Autodesk Inventor part; units mm, degrees
ref_plane "YZ Plane" through (0, 0, 0) normal (1, 0, 0) x (0, 1, 0)
ref_plane "XZ Plane" through (0, 0, 0) normal (0, 1, 0) x (-1, 0, 0)
ref_plane "XY Plane" through (0, 0, 0) normal (0, 0, 1) x (1, 0, 0)
sketch "Sketch1" plane through (0, 0, 0) normal (0, 1, 0) x (-1, 0, 0)
  line L0 (0, 0) -> (33, 0)
  line L1 (33, 0) -> (33, -28)
  line L2 (33, -28) -> (0, -28)
  line L3 (0, -28) -> (0, 0)
  line L4 (0, -17.5) -> (-20, -17.5)
  line L5 (-20, -17.5) -> (-20, -10.5)
  line L6 (-20, -10.5) -> (0, -10.5)
  line L7 (0, -10.5) -> (0, -17.5)
  line L8 (33, -17.5) -> (53, -17.5)
  line L9 (53, -17.5) -> (53, -10.5)
  line L10 (53, -10.5) -> (33, -10.5)
  line L11 (33, -10.5) -> (33, -17.5)
  line L12 (20, -28) -> (13, -28)
  line L13 (13, -28) -> (13, -48)
  line L14 (13, -48) -> (20, -48)
  line L15 (20, -48) -> (20, -28)
  line L16 (20, 0) -> (13, 0)
  line L17 (13, 0) -> (13, 20)
  line L18 (13, 20) -> (20, 20)
  line L19 (20, 20) -> (20, 0)
  circle A0 centre (16.5, -44) radius 1.75
  circle A1 centre (-16, -14) radius 1.75
  circle A2 centre (16.5, 16) radius 1.75
  circle A3 centre (49, -14) radius 1.75
  line L20 (16.5, -44) -> (16.5, -48) construction
  line L21 (-16, -14) -> (-20, -14) construction
  line L22 (16.5, 16) -> (16.5, 20) construction
  line L23 (49, -14) -> (53, -14) construction
  circle A4 centre (43, -14) radius 1.75
  circle A5 centre (37, -14) radius 1.75
  circle A6 centre (16.5, -38) radius 1.75
  circle A7 centre (16.5, -32) radius 1.75
  circle A8 centre (-10, -14) radius 1.75
  circle A9 centre (-4, -14) radius 1.75
  circle A10 centre (16.5, 10) radius 1.75
  circle A11 centre (16.5, 4) radius 1.75
  point P0 (16.5, -28)
  point P1 (16.5, 0)
  point P2 (0, -14)
  point P3 (33, -14)
  dimension "d0" = 33
  dimension "d1" = 28
  dimension "d29" = 7
  dimension "d34" = 20
  dimension "d35" = 4
  dimension "d36" = 3.5
  dimension "d44" = 6
  dimension "d51" = 6
  dimension "d58" = 6
  dimension "d65" = 6
extrude "Extrusion1" add sketch "Sketch1" along normal blind 2
sketch "Sketch2" plane through (0, 2, 0) normal (0, 1, 0) x (1, 0, 0)
  line L0 (0, 28) -> (-13, 28)
  line L1 (-33, 28) -> (-33, 17.5)
  line L2 (-33, 0) -> (-20, 0)
  line L3 (0, 0) -> (0, 10.5)
  line L4 (-26.6, 1.85) -> (-6.4, 1.85)
  line L5 (-6.4, 1.85) -> (-6.4, 4.05)
  line L6 (-6.4, 4.05) -> (-26.6, 4.05)
  line L7 (-26.6, 4.05) -> (-26.6, 1.85)
  line L8 (-26.6, 23.95) -> (-6.4, 23.95)
  line L9 (-6.4, 23.95) -> (-6.4, 26.15)
  line L10 (-6.4, 26.15) -> (-26.6, 26.15)
  line L11 (-26.6, 26.15) -> (-26.6, 23.95)
  line L12 (-26.6, 1.85) -> (-33, 1.85)
  line L13 (-26.6, 1.85) -> (-26.6, 0)
  line L14 (-26.6, 26.15) -> (-26.6, 28)
  line L15 (-6.4, 4.05) -> (0, 4.05)
  line L16 (-13, 28) -> (-13, 48)
  line L17 (-13, 48) -> (-20, 48)
  line L18 (-20, 48) -> (-20, 28)
  line L19 (-20, 28) -> (-33, 28)
  line L20 (-33, 17.5) -> (-53, 17.5)
  line L21 (-53, 17.5) -> (-53, 10.5)
  line L22 (-53, 10.5) -> (-33, 10.5)
  line L23 (-33, 10.5) -> (-33, 0)
  line L24 (-20, 0) -> (-20, -20)
  line L25 (-20, -20) -> (-13, -20)
  line L26 (-13, -20) -> (-13, 0)
  line L27 (-13, 0) -> (0, 0)
  line L28 (0, 10.5) -> (20, 10.5)
  line L29 (20, 10.5) -> (20, 17.5)
  line L30 (20, 17.5) -> (0, 17.5)
  line L31 (0, 17.5) -> (0, 28)
  line L32 (-28.5, 21.5) -> (-4.5, 21.5)
  line L33 (-4.5, 21.5) -> (-4.5, 6.5)
  line L34 (-4.5, 6.5) -> (-28.5, 6.5)
  line L35 (-28.5, 6.5) -> (-28.5, 21.5)
  line L36 (-28.5, 21.5) -> (-4.5, 6.5) construction
  line L37 (-4.5, 21.5) -> (-28.5, 6.5) construction
  point P0 (-16.5, 14)
  point P1 (-16.5, 23.95)
  point P2 (20, 14)
  dimension "d4" = 2.2
  dimension "d5" = 20.2
  dimension "d6" = 19.9
  dimension "d37" = 24
  dimension "d38" = 15
extrude "Extrusion2" cut sketch "Sketch2" against normal through all contours L10 L9 L8 L11 | L5 L4 L7 L6 | L32 L33 L34 L35
fillet "Fillet1" radius 3.5 8 edges at (-20, 1, 20) (-13, 1, 20) (20, 1, -10.5) (20, 1, -17.5) (-13, 1, -48) (-20, 1, -48) (-53, 1, -17.5) (-53, 1, -10.5)
fillet "Fillet2" radius 7 4 edges at (-33, 1, 0) (-33, 1, -28) (0, 1, -28) (0, 1, 0)
fillet "Fillet3" radius 2 4 edges at (-28.5, 1, -21.5) (-4.5, 1, -21.5) (-28.5, 1, -6.5) (-4.5, 1, -6.5)
sketch "Sketch4" plane through (0, 2, 0) normal (0, 1, 0) x (1, 0, 0)
  arc A0 (-4.5, 19.5) -> (-6.5, 21.5) centre (-6.5, 19.5) ccw construction
  line L0 (-26.5, 21.5) -> (-6.5, 21.5) construction
  line L1 (-4.5, 19.5) -> (-4.5, 8.5) construction
  arc A1 (-6.5, 6.5) -> (-4.5, 8.5) centre (-6.5, 8.5) ccw construction
  line L2 (-6.5, 6.5) -> (-26.5, 6.5) construction
  arc A2 (-28.5, 8.5) -> (-26.5, 6.5) centre (-26.5, 8.5) ccw construction
  line L3 (-28.5, 8.5) -> (-28.5, 19.5) construction
  arc A3 (-26.5, 21.5) -> (-28.5, 19.5) centre (-26.5, 19.5) ccw construction
  line L4 (-25.5, 21.5) -> (-23.5, 21.5)
  line L5 (-23.5, 21.5) -> (-23.5, 6.5)
  line L6 (-23.5, 6.5) -> (-25.5, 6.5)
  line L7 (-25.5, 6.5) -> (-25.5, 21.5)
  line L8 (-9.5, 6.5) -> (-7.5, 6.5)
  line L9 (-7.5, 6.5) -> (-7.5, 21.5)
  line L10 (-7.5, 21.5) -> (-9.5, 21.5)
  line L11 (-9.5, 21.5) -> (-9.5, 6.5)
  point P0 (0, 0)
  dimension "d70" = 3
  dimension "d71" = 3
  dimension "d72" = 2
properties part number "SoporteMarkers12"
Here's how the part is built. I have some questions about the finished solid (model axes, mm). A direction names the side the tool comes from. Round coordinates to 2 decimals unless told otherwise and drop trailing zeros. Order: outer loops, then holes, each group sorted by start corner. A loop starts at its lowest first (then second) coordinate and runs counter-clockwise, first axis right, second up. Notation, with made-up numbers: M 17,16 L 34,16 A22 ccw 34,28 Z; hole C 22.25,9 d2. An arc over 180 degrees is marked long. Use CSV: the item, a comma, the result in double quotes.
1) I want a section at A-A (x = -10.5). List the corners of the cut face in (y, z) for me.
Taken from the geometry:
outline,"M 0,-28 L 2,-28 L 2,-26.15 L 0,-26.15 Z; M 0,-23.95 L 2,-23.95 L 2,-21.5 L 0,-21.5 Z; M 0,-6.5 L 2,-6.5 L 2,-4.05 L 0,-4.05 Z; M 0,-1.85 L 2,-1.85 L 2,0 L 0,0 Z"
2) If we mould it in two halves opening along Z, with no side actions, what happens to faces 5 (the cylindrical face through (-16.12, 0.99, -42.29)), 6 (the flat face through (-33, 1, -9)), 7 (the cylindrical face through (-31, 1, -2.1))? For each: pulls with the +Z half, pulls with the -Z half, needs draft (parallel to the pull), parting line crosses it, or undercut.
Taken from the geometry:
face 5,"undercut"
face 6,"needs draft"
face 7,"pulls with the +Z half"
3) I want a section at D-D (y = 1.1). Count the separate pieces of the cut face and the enclosed holes in it, then the cut area to 3 significant figures.
Taken from the geometry:
separate pieces,"1"
enclosed holes,"15"
area,"860 mm^2"
4) I want a section at C-C (x = 4). List the corners of the cut face in (y, z) for me, then the cut area to 3 significant figures.
Taken from the geometry:
outline,"M 0,-17.5 L 2,-17.5 L 2,-15.75 L 0,-15.75 Z; M 0,-12.25 L 2,-12.25 L 2,-10.5 L 0,-10.5 Z"
area,"7.00 mm^2"
5) I'm going to push flat-ended pins straight in: P1, Ø0.6, axis at y = 1, z = -12, coming from the +X side; P2, Ø4.5, axis at x = -16.5, z = -32, coming from the +Y side; P3, Ø1, axis at y = 1.5, z = -25, coming from the -X side; P4, Ø3, axis at x = -16.5, z = 4, coming from the +Y side. Where does each tip first touch, or does it pass through?
Taken from the geometry:
P1,"x = 19.56"
P2,"y = 2"
P3,"x = -32.06"
P4,"through"
6) I want a section at B-B (z = -38). List the corners of the cut face in (x, y) for me.
Taken from the geometry:
outline,"M -20,0 L -18.25,0 L -18.25,2 L -20,2 Z; M -14.75,0 L -13,0 L -13,2 L -14.75,2 Z"
7) On a 3-axis mill with a long thin cutter (end or side, diameter ignored), from which of +Z, -Z, +X, -X, +Y, -Y can I reach the whole of each face in a straight line? I mean faces 1 (the flat face through (-10, 1, -28)), 2 (the flat face through (-28.5, 1, -14)), 3 (the flat face through (-41, 1, -17.5)), 4 (the cylindrical face through (-2.1, 1, -2)). Say none if no direction works.
Taken from the geometry:
face 1,"-Z, +X, +Y, -Y"
face 2,"+Y, -Y"
face 3,"-Z, -X, +Y, -Y"
face 4,"+Z, +X, +Y, -Y"
8) I need wall thicknesses on line 1 along X through (y, z) = (1.3, -18); line 2 along Z through (x, y) = (-43, 0.75); line 3 along X through (y, z) = (1.6, -35). Which ranges of each line are inside material? Lowest first, please. Write a range as [from, to].
Taken from the geometry:
line 1,"[-33, -28.5], [-4.5, 0]"
line 2,"[-17.5, -15.75], [-12.25, -10.5]"
line 3,"[-20, -13]"
